from build123d import *

# Parameters (mm, degrees)
SKETCH1_R           = 6.35
BOSS_EXTRUDE1_DEPTH = 508
SKETCH2_W           = 3.175
SKETCH2_H           = 3.175
CUT_EXTRUDE1_DEPTH  = 38.1
SKETCH3_R           = 9.19467987
SKETCH3_R_2         = 5.9436
CUT_EXTRUDE2_DEPTH  = 0.9906
CHAMFER1_SIZE       = 0.254
FILLET1_R           = 1.5875


with BuildPart() as part:
    # Sketch1 → Boss-Extrude1 (new body)
    with BuildSketch(Plane.XY):
        Circle(SKETCH1_R)
    extrude(amount=BOSS_EXTRUDE1_DEPTH)

    # Sketch2 → Cut-Extrude1 (cut)
    with BuildSketch(Plane(origin=(0, 0, 0), x_dir=(-1, 0, 0), z_dir=(0, 0, -1))):
        with Locations((0, 6.35)):
            Rectangle(SKETCH2_W, SKETCH2_H)
    extrude(amount=-CUT_EXTRUDE1_DEPTH, mode=Mode.SUBTRACT)

    # Sketch3 → Cut-Extrude2 (cut)
    with BuildSketch(Plane(origin=(0, 0, 3.175), x_dir=(-1, 0, 0), z_dir=(0, 0, -1))):
        Circle(SKETCH3_R)
        Circle(SKETCH3_R_2, mode=Mode.SUBTRACT)
    extrude(amount=-CUT_EXTRUDE2_DEPTH, mode=Mode.SUBTRACT)

    # Chamfer1
    chamfer1_edges = [part.edges().sort_by_distance(p)[0] for p in [
        (0, -6.35, 0),
    ]]
    chamfer(chamfer1_edges, length=CHAMFER1_SIZE)

    # Fillet1
    fillet1_edges = [part.edges().sort_by_distance(p)[0] for p in [
        (-1.5875, 5.455430531, 38.1),
        (1.5875, 5.455430531, 38.1),
    ]]
    fillet(fillet1_edges, radius=FILLET1_R - 0.0001)  # a hair under: the kernel refuses the full size


solid = part.part
Could you check a few things on this model? Use its own coordinates, in mm. A direction names the side the tool comes from. Give positions to 0.01 mm unless a question says otherwise; leave off trailing zeros. Write each loop counter-clockwise with the first axis right and the second up, starting at its lowest first coordinate (ties: lowest second). Pieces come first, ordered by that corner, then holes. Notation, with made-up numbers: (12, -25) -> (33, -25) arc R17 ccw to (33, -8) -> close; hole circle Ø11 at (35.5, 74). An arc over 180 degrees is marked (long way). Answer as CSV lines item,"result". Start each with the question number.
(1) If we mould it in two halves opening along Z, with no side actions, what happens to faces 1 (the face through (-0.257, -6.345, 1.694)), 2 (the face through (-0.25, -6.22, 0.13)), 3 (the face through (0, -6.1, 4.166))? For each: +Z half, -Z half, draft (parallel to the pull), parting line (faces both ways), or undercut.
(2) Which directions (+Z, -Z, +X, -X, +Y, -Y) give clear straight access to the entire face, cutting with the end or side of a thin tool? Please do faces 4 (the face through (0, 0, 0)), 5 (the face through (0, -6.1, 3.175)).
(3) If we section it at A-A, the plane z = 381: Write out the boundary of the cut face in (x, y).
(4) I'm going to push flat-ended pins straight in: pin 1 Ø1 at (y, z) = (-4.5, 326) entering from +X; pin 2 Ø1.1 at (y, z) = (5.5, 15.5) entering from -X; pin 3 Ø1 at (y, z) = (2, 223) entering from +X. Where does each tip first touch, or does it pass through?
(5) Please list where these lines run through material, in increasing order: line 1 (X direction, y = -1, z = 292.5); line 2 (Y direction, x = 0.75, z = 357); line 3 (Y direction, x = 1.5, z = 51).
Answer list:
1,face 1,"draft"
1,face 2,"-Z half"
1,face 3,"undercut"
2,face 4,"-Z, +X, -X, +Y, -Y"
2,face 5,"none"
3,outline,"circle Ø12.7 at (0, 0)"
4,pin 1,"x = 4.93"
4,pin 2,"x = -3.98"
4,pin 3,"x = 6.17"
5,line 1,"-6.27 to 6.27"
5,line 2,"-6.31 to 6.31"
5,line 3,"-6.17 to 6.17"
